Read the model definition and answer for the solid it produces. Units are mm, in the model's axes. A direction names the side the tool comes from. Coordinates: 2 decimals unless noted, no trailing zeros. Write each loop counter-clockwise with the first axis right and the second up, starting at its lowest first coordinate (ties: lowest second). Pieces come first, ordered by that corner, then holes. Notation, with made-up numbers: (-11, 29) -> (43, 29) arc R34 ccw to (43, 64) -> close; hole circle Ø10 at (45.5, 38.25). An arc over 180 degrees is marked (long way). Use CSV: the item, a comma, the result in double quotes.
from build123d import *

# Parameters (mm, degrees)
SKETCH_1_W                 = 126
SKETCH_1_H                 = 126
EXTRUDE_2_DEPTH            = 40
SKETCH_7_W                 = 120
SKETCH_7_H                 = 120
CUT_EXTRUDE_1_DEPTH        = 35
EXTRUDE_3_OUTLINE_W        = 66
EXTRUDE_3_OUTLINE_H        = 66
EXTRUDE_3_OUTLINE_W_2      = 60
EXTRUDE_3_OUTLINE_H_2      = 60
EXTRUDE_3_DEPTH            = 35
EXTRUDE_3_2_OUTLINE_W      = 60
EXTRUDE_3_2_OUTLINE_H      = 60
EXTRUDE_3_2_DEPTH          = 3
EXTRUDE_START              = 32
EXTRUDE_3_3_OUTLINE_W      = 60
EXTRUDE_3_3_OUTLINE_H      = 60
EXTRUDE_3_3_DEPTH          = 3
SKETCH_9_W                 = 56
SKETCH_9_H                 = 20
CUT_EXTRUDE_2_DEPTH        = 3
SKETCH_10_W                = 100
SKETCH_10_H                = 100
SKETCH_10_W_2              = 98
SKETCH_10_H_2              = 98
EXTRUDE_3_4_DEPTH          = 10
SKETCH_11_R                = 3
CUT_EXTRUDE_3_DEPTH        = 3
SCALE_1_SCALE              = 1.666667
SKETCH_13_W                = 201.00004
SKETCH_13_H                = 201.00004
SKETCH_13_W_2              = 200.00004
SKETCH_13_H_2              = 200.00004
CUT_EXTRUDE_4_DEPTH        = 60
SKETCH_14_W                = 93.333352
SKETCH_14_H                = 15.000005
CUT_EXTRUDE_5_DEPTH        = 60
PATTERN_START              = -17.686023251
PATTERN_LINEAR_2_OUTLINE_R = 5.000001
PATTERN_LINEAR_2_DEPTH     = 5.000001
PATTERN_LINEAR_3_OUTLINE_R = 5.000001
PATTERN_LINEAR_3_DEPTH     = 5.000001
SKETCH_15_R                = 7.5
CUT_EXTRUDE_6_DEPTH        = 30


# Read off the part's stored shape, not the designer's step: 拉伸-薄壁3, 阵列(线性)2, 阵列(线性)3
with BuildPart() as part:
    # 草图1 → 凸台-拉伸2 (new body)
    with BuildSketch(Plane(origin=(0, 0, 0), x_dir=(1, 0, 0), z_dir=(0, 1, 0))):
        with Locations((63, -63)):
            Rectangle(SKETCH_1_W, SKETCH_1_H)
    extrude(amount=EXTRUDE_2_DEPTH)

    # 草图7 → 切除-拉伸1 (cut)
    with BuildSketch(Plane(origin=(0, 0, 0), x_dir=(1, 0, 0), z_dir=(0, 1, 0))):
        with Locations((63, -63)):
            Rectangle(SKETCH_7_W, SKETCH_7_H)
    extrude(amount=CUT_EXTRUDE_1_DEPTH, mode=Mode.SUBTRACT)

    # Extrude 3 outline → Extrude 3 (add)
    with BuildSketch(Plane.XZ.offset(-35)):
        with Locations((63, 63)):
            Rectangle(EXTRUDE_3_OUTLINE_W, EXTRUDE_3_OUTLINE_H)
        with Locations((63, 63)):
            Rectangle(EXTRUDE_3_OUTLINE_W_2, EXTRUDE_3_OUTLINE_H_2, mode=Mode.SUBTRACT)
    extrude(amount=EXTRUDE_3_DEPTH)

    # Extrude 3 2 outline → Extrude 3 2 (add)
    with BuildSketch(Plane.XZ.offset(-35)):
        with Locations((63, 63)):
            Rectangle(EXTRUDE_3_2_OUTLINE_W, EXTRUDE_3_2_OUTLINE_H)
    extrude(amount=EXTRUDE_3_2_DEPTH)

    # Extrude 3 3 outline → Extrude 3 3 (add)
    with BuildSketch(Plane.XZ.offset(-35).offset(EXTRUDE_START)):
        with Locations((63, 63)):
            Rectangle(EXTRUDE_3_3_OUTLINE_W, EXTRUDE_3_3_OUTLINE_H)
    extrude(amount=EXTRUDE_3_3_DEPTH)

    # 草图9 → 切除-拉伸2 (cut)
    with BuildSketch(Plane.XY.offset(96)):
        with Locations((64, 25)):
            Rectangle(SKETCH_9_W, SKETCH_9_H)
    extrude(amount=-CUT_EXTRUDE_2_DEPTH, mode=Mode.SUBTRACT)

    # 草图10 → Extrude 3 4 (add)
    with BuildSketch(Plane.XZ.offset(-35)):
        with Locations((63, 63)):
            Rectangle(SKETCH_10_W, SKETCH_10_H)
        with Locations((63, 63)):
            Rectangle(SKETCH_10_W_2, SKETCH_10_H_2, mode=Mode.SUBTRACT)
    extrude(amount=EXTRUDE_3_4_DEPTH)

    # 草图11 → 切除-拉伸3 (cut)
    with BuildSketch(Plane.XZ):
        with Locations(Location((50, 76, 0), (0, 0, 270))):
            Circle(SKETCH_11_R)
        with Locations(Location((76, 76, 0), (0, 0, 90))):
            Circle(SKETCH_11_R)
        with Locations(Location((76, 50, 0), (0, 0, 270))):
            Circle(SKETCH_11_R)
        with Locations(Location((50, 50, 0), (0, 0, 90))):
            Circle(SKETCH_11_R)
        with Locations(Location((63, 63, 0), (0, 0, 270))):
            Circle(SKETCH_11_R)
    extrude(amount=-CUT_EXTRUDE_3_DEPTH, mode=Mode.SUBTRACT)


with BuildPart() as part_1:
    # 缩放比例1: scaled about (62.981257937, 26.529021612, 62.409625003)
    add(part.part.scale(SCALE_1_SCALE).moved(Location((-41.987526285, -17.686023251, -41.606437472))))

    # 草图13 → 切除-拉伸4 (cut)
    with BuildSketch(Plane.XZ.offset(17.686023251)):
        with Locations((63.012494715, 63.393583528)):
            Rectangle(SKETCH_13_W, SKETCH_13_H)
        with Locations((63.012494715, 63.393583528)):
            Rectangle(SKETCH_13_W_2, SKETCH_13_H_2, mode=Mode.SUBTRACT)
    extrude(amount=-CUT_EXTRUDE_4_DEPTH, mode=Mode.SUBTRACT)

    # 草图14 → 切除-拉伸5 (cut)
    with BuildSketch(Plane.XY.offset(118.393594528)):
        with Locations((64.679161715, -0.186020751)):
            Rectangle(SKETCH_14_W, SKETCH_14_H)
    extrude(amount=-CUT_EXTRUDE_5_DEPTH, mode=Mode.SUBTRACT)

    # 阵列(线性)2 outline → 阵列(线性)2 (cut)
    with BuildSketch(Plane(origin=(0, 0, 0), x_dir=(1, 0, 0), z_dir=(0, 1, 0)).offset(PATTERN_START)):
        with Locations((63.012494715, -43.393583528)):
            Circle(PATTERN_LINEAR_2_OUTLINE_R)
        with Locations((41.345823715, -65.060254528)):
            Circle(PATTERN_LINEAR_2_OUTLINE_R)
        with Locations((84.679165715, -65.060254528)):
            Circle(PATTERN_LINEAR_2_OUTLINE_R)
        with Locations((84.679165715, -21.726912528)):
            Circle(PATTERN_LINEAR_2_OUTLINE_R)
        with Locations((41.345823715, -21.726912528)):
            Circle(PATTERN_LINEAR_2_OUTLINE_R)
    extrude(amount=PATTERN_LINEAR_2_DEPTH, mode=Mode.SUBTRACT)

    # 阵列(线性)3 outline → 阵列(线性)3 (cut)
    with BuildSketch(Plane(origin=(0, 0, 0), x_dir=(1, 0, 0), z_dir=(0, 1, 0)).offset(PATTERN_START)):
        with Locations((63.012494715, -86.293583528)):
            Circle(PATTERN_LINEAR_3_OUTLINE_R)
        with Locations((63.012494715, -106.293583528)):
            Circle(PATTERN_LINEAR_3_OUTLINE_R)
        with Locations((41.345823715, -107.960254528)):
            Circle(PATTERN_LINEAR_3_OUTLINE_R)
        with Locations((84.679165715, -107.960254528)):
            Circle(PATTERN_LINEAR_3_OUTLINE_R)
        with BuildLine():
            ThreePointArc((89.674469878, -64.843583528), (84.679165715, -59.626911528), (79.683861552, -64.843583528))
            ThreePointArc((79.683861552, -64.843583528), (84.679165715, -60.060253528), (89.674469878, -64.843583528))
        make_face()
        with BuildLine():
            ThreePointArc((89.674469878, -84.843583528), (84.679165715, -79.626911528), (79.683861552, -84.843583528))
            ThreePointArc((79.683861552, -84.843583528), (84.679165715, -80.060253528), (89.674469878, -84.843583528))
        make_face()
        with BuildLine():
            ThreePointArc((46.341127878, -64.843583528), (41.345823715, -59.626911528), (36.350519552, -64.843583528))
            ThreePointArc((36.350519552, -64.843583528), (41.345823715, -60.060253528), (46.341127878, -64.843583528))
        make_face()
        with BuildLine():
            ThreePointArc((46.341127878, -84.843583528), (41.345823715, -79.626911528), (36.350519552, -84.843583528))
            ThreePointArc((36.350519552, -84.843583528), (41.345823715, -80.060253528), (46.341127878, -84.843583528))
        make_face()
    extrude(amount=PATTERN_LINEAR_3_DEPTH, mode=Mode.SUBTRACT)

    # 草图15 → 切除-拉伸6 (cut)
    with BuildSketch(Plane.XZ.offset(17.686023251)):
        with Locations(Location((103.012505715, 68.393594528, 0), (0, 0, 270))):
            Circle(SKETCH_15_R)
        with Locations(Location((23.012483715, 68.393594528, 0), (0, 0, 270))):
            Circle(SKETCH_15_R)
    extrude(amount=-CUT_EXTRUDE_6_DEPTH, mode=Mode.SUBTRACT)


solid = part_1.part
1. A tool of negligible diameter and unlimited length cuts with its end or side. For faces 1 (the flat face through (113.013, 12, 63)), 2 (the flat face through (163.513, 12, 62)), from which of +Z, -Z, +X, -X, +Y, -Y can it reach the whole face along a straight path? Write none if from no direction.
Solutions:
face 1,"none"
face 2,"-Y"
2. A cutting plane is placed at A-A (y = 29). Give the vertices of the cut face in (x, z).
Solutions:
outline,"(-41.99, -41.61) -> (168.01, -41.61) -> (168.01, 168.39) -> (-41.99, 168.39) -> close; (-20.32, -19.94) -> (146.35, -19.94) -> (146.35, 146.73) -> (-20.32, 146.73) -> close; (8.01, 8.39) -> (118.01, 8.39) -> (118.01, 118.39) -> (111.35, 118.39) -> (111.35, 113.39) -> (113.01, 113.39) -> (113.01, 13.39) -> (13.01, 13.39) -> (13.01, 113.39) -> (18.01, 113.39) -> (18.01, 118.39) -> (8.01, 118.39) -> close; hole (-37.49, -37.11) -> (163.51, -37.11) -> (163.51, 163.89) -> (-37.49, 163.89) -> close; hole (-18.65, -18.27) -> (144.68, -18.27) -> (144.68, 145.06) -> (-18.65, 145.06) -> close"
3. A cutting plane is placed at B-B (y = 3). Give the vertices of the cut face in (x, z), and give its area (3 significant figures).
Solutions:
outline,"(-41.99, -41.61) -> (168.01, -41.61) -> (168.01, 168.39) -> (-41.99, 168.39) -> close; (8.01, 8.39) -> (118.01, 8.39) -> (118.01, 118.39) -> (111.35, 118.39) -> (111.35, 113.39) -> (113.01, 113.39) -> (113.01, 13.39) -> (13.01, 13.39) -> (13.01, 113.39) -> (18.01, 113.39) -> (18.01, 118.39) -> (8.01, 118.39) -> close; hole (-37.49, -37.11) -> (163.51, -37.11) -> (163.51, 163.89) -> (-37.49, 163.89) -> close"
area,"5,330 mm^2"
4. For a pull along X with two mould halves and no side action, classify faces 3 (the flat face through (-41.988, 15, 65)), 4 (the flat face through (-37.488, 12, 62)), 5 (the flat face through (-39, -17.686, 63)) as pulls with the +X half, pulls with the -X half, needs draft (parallel to the pull), parting line crosses it, or undercut.
Solutions:
face 3,"pulls with the -X half"
face 4,"undercut"
face 5,"needs draft"
5. A cutting plane is placed at D-D (z = -9). Give the vertices of the cut face in (x, y).
Solutions:
outline,"(-41.99, -17.69) -> (-37.49, -17.69) -> (-37.49, 42.31) -> (-36.99, 42.31) -> (-36.99, 40.65) -> (-20.32, 40.65) -> (-20.32, 23.98) -> (-18.65, 23.98) -> (-18.65, 40.65) -> (144.68, 40.65) -> (144.68, 23.98) -> (146.35, 23.98) -> (146.35, 40.65) -> (163.01, 40.65) -> (163.01, 42.31) -> (163.51, 42.31) -> (163.51, -17.69) -> (168.01, -17.69) -> (168.01, 48.98) -> (-41.99, 48.98) -> close"
6. Find the intervals of material crossed by line 1 along Z through (x, y) = (21.5, 32.5); line 2 along X through (y, z) = (0, 18); line 3 along X through (y, z) = (18.5, 11.5), in increasing order.
Solutions:
line 1,"z = -41.61 to -37.11, -19.94 to -18.27, 8.39 to 13.39, 145.06 to 146.73, 163.89 to 168.39"
line 2,"x = -41.99 to -37.49, 8.01 to 13.01, 113.01 to 118.01, 163.51 to 168.01"
line 3,"x = -41.99 to -37.49, 8.01 to 118.01, 163.51 to 168.01"
7. Each of these flat-tipped pins is pushed along its axis until it touches: pin 1 Ø8 at (x, z) = (84.68, 21.73) entering from -Y; pin 2 Ø2 at (x, z) = (-15, 23) entering from -Y. Where does it stop, or does it pass through?
Solutions:
pin 1,"stops at y = 35.65"
pin 2,"stops at y = 40.65"
